```python
from build123d import *

# Parameters (mm, degrees)
BASE_WALL_DEPTH     = 70
BASE_SUPPORT_START  = -61.5
BASE_SUPPORT_DEPTH  = 61.5
SKETCH4_W           = 8
SKETCH4_H           = 30
MOUNT_NOTCH_DEPTH   = 61.5
SKETCH5_R           = 1.65
SCREW_HOLE_M3_DEPTH = 181.5
SKETCH6_W           = 8
SKETCH6_H           = 30
CUT_EXTRUDE4_DEPTH  = 181.5
SKETCH7_R           = 1.65
CUT_EXTRUDE5_DEPTH  = 181.5


with BuildPart() as part:
    # Sketch1 → Base_Wall (new body)
    with BuildSketch(Plane(origin=(0, 0, 0), x_dir=(1, 0, 0), z_dir=(0, 1, 0))):
        with BuildLine():
            Line((75, 0), (90.075, 0))
            ThreePointArc((90.075, 0), (63.692643315, -63.692643315), (0, -90.075))
            Line((0, -90.075), (0, -75))
            ThreePointArc((0, -75), (53.033008589, -53.033008589), (75, 0))
        make_face()
    extrude(amount=BASE_WALL_DEPTH)

    # Sketch3 → Base_Support (add)
    with BuildSketch(Plane(origin=(0, 70, 0), x_dir=(1, 0, 0), z_dir=(0, 1, 0)).offset(BASE_SUPPORT_START)):
        with BuildLine():
            Line((0, -75), (0, -60))
            ThreePointArc((0, -60), (42.426406871, -42.426406871), (60, 0))
            Line((60, 0), (75, 0))
            ThreePointArc((75, 0), (53.033008589, -53.033008589), (0, -75))
        make_face()
    extrude(amount=BASE_SUPPORT_DEPTH)

    # Sketch4 → Mount-Notch (cut)
    with BuildSketch(Plane(origin=(0, 0, 0), x_dir=(-1, 0, 0), z_dir=(0, 0, -1))):
        with Locations((-90.075, 39.25)):
            Rectangle(SKETCH4_W, SKETCH4_H)
    extrude(amount=-MOUNT_NOTCH_DEPTH, mode=Mode.SUBTRACT)

    # Sketch5 → Screw-Hole-M3 (cut)
    with BuildSketch(Plane(origin=(0, 0, 0), x_dir=(0, 0, -1), z_dir=(1, 0, 0))):
        with Locations(Location((-13.272151295, 39.25, 0), (0, 0, 180))):
            Circle(SKETCH5_R)
    extrude(amount=SCREW_HOLE_M3_DEPTH, mode=Mode.SUBTRACT)

    # Sketch6 → Cut-Extrude4 (cut)
    with BuildSketch(Plane.ZY):
        with Locations((90.075, 39.294262642)):
            Rectangle(SKETCH6_W, SKETCH6_H)
    extrude(amount=-CUT_EXTRUDE4_DEPTH, mode=Mode.SUBTRACT)

    # Sketch7 → Cut-Extrude5 (cut)
    with BuildSketch(Plane.XY.offset(86.075)):
        with Locations((13.272151295, 39.294262642)):
            Circle(SKETCH7_R)
    extrude(amount=-CUT_EXTRUDE5_DEPTH, mode=Mode.SUBTRACT)


solid = part.part
```
Work out the finished part from the listing and answer in its coordinate system (mm). A direction names the side the tool comes from. Round coordinates to 2 decimals unless told otherwise and drop trailing zeros. Order: outer loops, then holes, each group sorted by start corner. A loop starts at its lowest first (then second) coordinate and runs counter-clockwise, first axis right, second up.
Q1. A cutting plane is placed at A-A, the plane x = 65.5. Determine the outline of the cut face in (y, z), then the cut area to 3 significant figures.
Solution:
outline: (0, 36.53) - (8.5, 36.53) - (8.5, 0) - (70, 0) - (70, 61.83) - (0, 61.83) - close; hole circle Ø3.3 at (39.25, 13.27)
area: 4,010 mm2
Q2. A cutting plane is placed at C-C, the plane y = 26.5. Determine the outline of the cut face in (x, z) (3 decimals), then the cut area to 3 significant figures.
Solution:
outline: (0, 60) arc R60 cw to (60, 0) - (86.075, 0) - (86.075, 26.544) arc R90.075 ccw to (26.544, 86.075) - (0, 86.075) - close
area: 3,400 mm2
Q3. Given pin 1 Ø8 at (x, y) = (19, 46) entering from +Z (3 decimals); pin 2 Ø6 at (y, z) = (33, 13) entering from +X (3 decimals); pin 3 Ø1 at (x, y) = (68.5, 16) entering from +Z, each flat-ended and moving along its own axis, determine where each tip first touches the part or whether it passes through.
Solution:
pin 1: stops at z = 86.075
pin 2: stops at x = 86.075
pin 3: stops at z = 59.07
Q4. A cutting plane is placed at B-B, the plane z = 7. Determine the outline of the cut face in (x, y) (3 decimals), then the cut area to 3 significant figures.
Solution:
outline: (59.59, 8.5) - (74.673, 8.5) - (74.673, 0) - (89.803, 0) - (89.803, 24.25) - (86.075, 24.25) - (86.075, 54.25) - (89.803, 54.25) - (89.803, 70) - (59.59, 70) - close
area: 1,870 mm2
Q5. A tool of negligible diameter and unlimited length cuts with its end or side. For faces 4 (the cylindrical face through (52.45, 4.19, 53.61)), 5 (the flat face through (10, 39, 86.075)), 6 (the flat face through (88, 54.25, 10)), 7 (the flat face through (0, 35, 75)), 8 (the flat face through (75, 35, 0)), from which of +Z, -Z, +X, -X, +Y, -Y can it reach the whole face along a straight path? Write none if from no direction.
Solution:
face 4: -Z, -X, -Y
face 5: +Z, +X, -X
face 6: +Z, -Z, +X
face 7: +Z, -Z, -X, +Y, -Y
face 8: -Z, +X, -X, +Y, -Y
Q6. The mould has two halves that part along Z. Classify faces 1 (the cylindrical face through (41.96, 38.82, 42.89)), 2 (the flat face through (86.075, 39, 10)), 3 (the cylindrical face through (71.9, 38.13, 12.06)): pulls with the +Z half, pulls with the -Z half, needs draft (parallel to the pull), parting line crosses it, or undercut.
Solution:
face 1: pulls with the -Z half
face 2: needs draft
face 3: undercut
Q7. A cutting plane is placed at D-D, the plane z = 80.5. Determine the outline of the cut face in (x, y), then the cut area to 3 significant figures.
Solution:
outline: (0, 0) - (40.41, 0) - (40.41, 70) - (0, 70) - close; hole circle Ø3.3 at (13.27, 39.29)
area: 2,820 mm2
Q8. Find the intervals of material crossed by line 1 along Y through (x, z) = (45, 45.5); line 2 along Z through (x, y) = (15, 24.5) (3 decimals); line 3 along Z through (x, y) = (68, 39.25), in increasing order.
Solution:
line 1: y = 8.5 to 70
line 2: z = 58.095 to 86.075
line 3: z = 0 to 11.62, 14.92 to 59.07
